Can you work these out from the model? Positions are in its coordinate system, mm. Face numbers are marked on the shaded views. Round coordinates to 2 decimals unless told otherwise and drop trailing zeros. Order: outer loops, then holes, each group sorted by start corner. A loop starts at its lowest first (then second) coordinate and runs counter-clockwise, first axis right, second up.
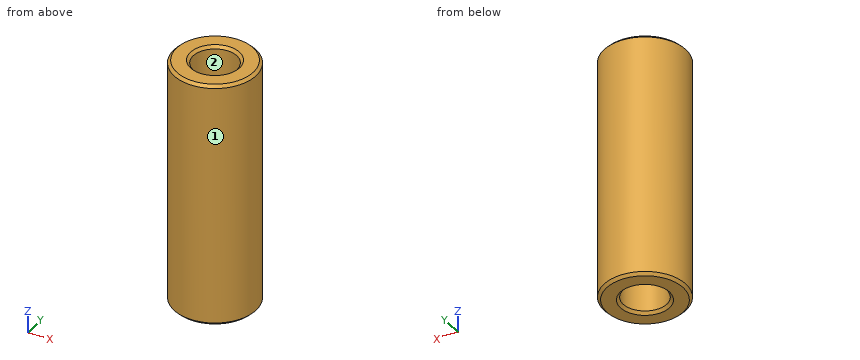
from build123d import *

# Parameters (mm, degrees)
SKETCH_1_R      = 7.5
SKETCH_1_R_2    = 4
EXTRUDE_1_DEPTH = 45
CHAMFER_1_SIZE  = 0.5


with BuildPart() as part:
    # Эскиз1 → Бобышка-Вытянуть1 (new body)
    with BuildSketch(Plane.XY):
        with Locations(Location((0, 0, 0), (0, 0, 180))):
            Circle(SKETCH_1_R)
        with Locations(Location((0, 0, 0), (0, 0, 180))):
            Circle(SKETCH_1_R_2, mode=Mode.SUBTRACT)
    extrude(amount=EXTRUDE_1_DEPTH)

    # Фаска1
    chamfer_1_edges = [part.edges().sort_by_distance(p)[0] for p in [
        (7.5, 0, 0),
        (7.5, 0, 45),
        (4, 0, 0),
        (4, 0, 45),
    ]]
    chamfer(chamfer_1_edges, length=CHAMFER_1_SIZE)


solid = part.part
(1) I want a section at A-A, the plane x = 0. List the corners of the cut face in (y, z) for me.
(2) I want a section at C-C, the plane z = 31.5. List the corners of the cut face in (x, y) for me.
(3) Please list where these lines run through material, in increasing order: probe 1 along Y at (x, z) = (0, 22); probe 2 along X at (y, z) = (-0.5, 20); probe 3 along X at (y, z) = (-2.25, 33).
(4) If we mould it in two halves opening along X, with no side actions, what happens to the marked faces 1 and 2? For each: pulls with the +X half, pulls with the -X half, needs draft (parallel to the pull), parting line crosses it, or undercut.
(5) I'm going to push flat-ended pins straight in: pin 1 Ø5 at (y, z) = (5.5, 9) entering from -X; pin 2 Ø1 at (y, z) = (-4, 24) entering from +X; pin 3 Ø3 at (y, z) = (-5.5, 27.5) entering from -X. Where does each tip first touch, or does it pass through?
Ans:
1. outline: (-7.5, 0.5) - (-7, 0) - (-4.5, 0) - (-4, 0.5) - (-4, 44.5) - (-4.5, 45) - (-7, 45) - (-7.5, 44.5) - close; (4, 0.5) - (4.5, 0) - (7, 0) - (7.5, 0.5) - (7.5, 44.5) - (7, 45) - (4.5, 45) - (4, 44.5) - close
2. outline: circle Ø15 at (0, 0); hole circle Ø8 at (0, 0)
3. probe 1: y = -7.5 to -4, 4 to 7.5
3. probe 2: x = -7.48 to -3.97, 3.97 to 7.48
3. probe 3: x = -7.15 to -3.31, 3.31 to 7.15
4. face 1: parting line crosses it
4. face 2: undercut
5. pin 1: stops at x = -6.87
5. pin 2: stops at x = 6.63
5. pin 3: stops at x = -6.34
